Study the drawing (mm; zero at the part's minimum x, y, z) and answer. A direction names the side the tool comes from. Coordinates: 2 decimals unless noted, no trailing zeros. Order: outer loops, then holes, each group sorted by start corner. A loop starts at its lowest first (then second) coordinate and runs counter-clockwise, first axis right, second up. Notation, with made-up numbers: M 65.25,-40 L 95.25,-40 A13 cw 95.25,-29 Z; hole C -36,58.25 d9. An arc over 180 degrees is marked long. One line per item, written item: value. Start each with the question number.
Q1. The part is cut by section D-D on y = 56.5. Give the vertices of the cut face in (x, z), then the cut area to 3 significant figures.
Q2. For the marked faces 5 and 6, determine the directions among +Z, -Z, +X, -X, +Y, -Y from which every point of the face is accessible in a straight line to the end or side of a thin tool.
Q3. Each of these flat-tipped pins is pushed along its axis until it touches: pin 1 Ø5 at (x, y) = (29.9, 29.9) entering from -Z; pin 2 Ø12 at (x, z) = (51.5, 18) entering from +Y; pin 3 Ø2 at (x, z) = (18, 25) entering from +Y; pin 4 Ø5 at (x, z) = (29, 5.5) entering from +Y. Where does it stop, or does it pass through?
Q4. Straight lines are drawn through the part: line 1 along Z through (x, y) = (11, 47); line 2 along Y through (x, z) = (29.9, 6.5); line 3 along Y through (x, z) = (6.5, 20.5). For each, find the intervals that lie inside material, in ascending order. Write a range as [from, to].
Q5. The part is cut by section A-A on x = 29.9. Give the vertices of the cut face in (y, z).
Q6. The part is cut by section C-C on z = 16.25. Give the vertices of the cut face in (x, y), then the cut area to 3 significant figures.
Q7. Determine the mould class of the marked faces 1, 2, 3 and 4 for opening direction Z: pulls with the +Z half, pulls with the -Z half, needs draft (parallel to the pull), parting line crosses it, or undercut.
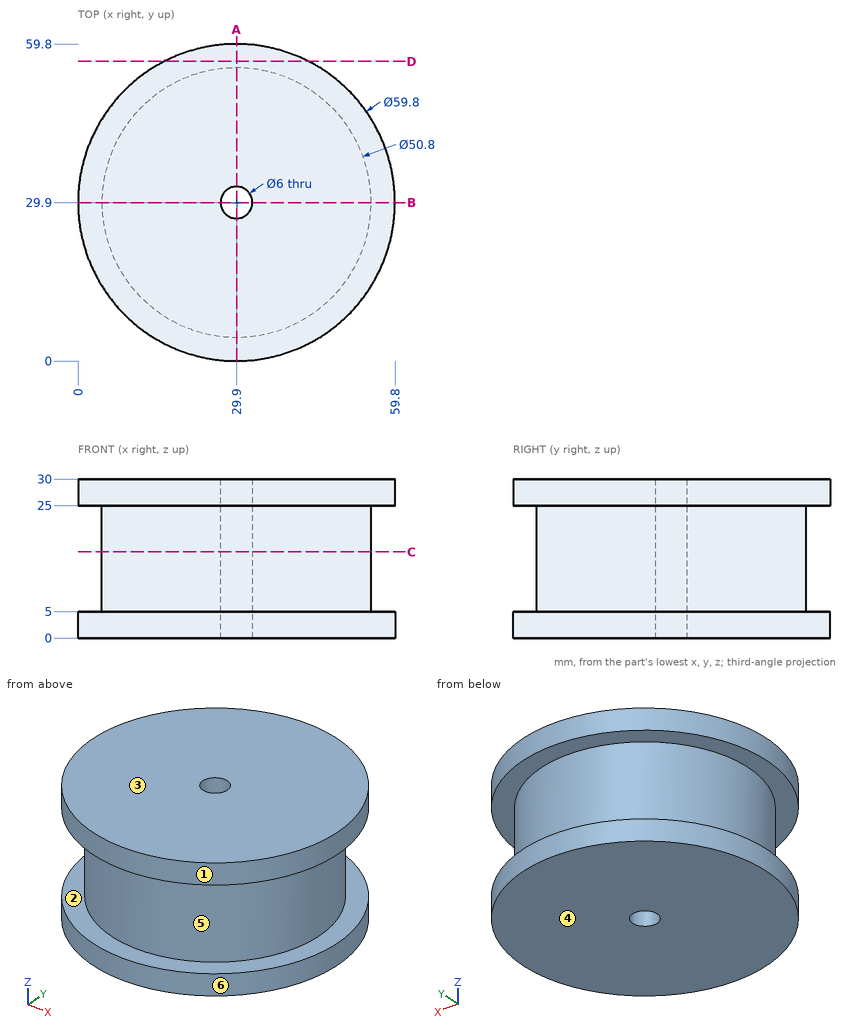
Output:
1. outline: M 16.25,0 L 43.55,0 L 43.55,5 L 16.25,5 Z; M 16.25,25 L 43.55,25 L 43.55,30 L 16.25,30 Z
1. area: 273 mm^2
2. face 5: none
2. face 6: +Z, -Z
3. pin 1: passes through
3. pin 2: stops at y = 49.94
3. pin 3: stops at y = 57.74
3. pin 4: stops at y = 59.8
4. line 1: z = [0, 5], [25, 30]
4. line 2: y = [4.5, 26.9], [32.9, 55.3]
4. line 3: y = [20.02, 39.78]
5. outline: M 0,0 L 26.9,0 L 26.9,30 L 0,30 L 0,25 L 4.5,25 L 4.5,5 L 0,5 Z; M 32.9,0 L 59.8,0 L 59.8,5 L 55.3,5 L 55.3,25 L 59.8,25 L 59.8,30 L 32.9,30 Z
6. outline: C 29.9,29.9 d50.8; hole C 29.9,29.9 d6
6. area: 2,000 mm^2
7. face 1: needs draft
7. face 2: undercut
7. face 3: pulls with the +Z half
7. face 4: pulls with the -Z half
